For this review, use the dimensioned drawing (mm, ordinates from the lowest corner) and the shaded views. A direction names the side the tool comes from. Coordinates: 2 decimals unless noted, no trailing zeros. Loops run counter-clockwise (first coordinate to the right, second up) from the corner with the lowest first, then second, coordinate; pieces in that order, holes last. Notation, with made-up numbers: (-29.5, 60) - (29.5, 60) arc R18 ccw to (29.5, 70) - close; hole circle Ø4 at (-21, 66). An arc over 180 degrees is marked (long way). Answer in a Markdown table with one row per item. Add a question column.
(1) For P1, Ø4.5, axis at x = 27.432, y = 15.748, coming from the -Z side; P2, Ø6, axis at x = 11.5, z = 5, coming from the +Y side; P3, Ø5, axis at x = 24.5, y = 14, coming from the -Z side; P4, Ø4, axis at x = 9.5, z = 2.5, coming from the +Y side, all flat-tipped, find the tip position at first contact; note any pin that passes through.
(2) For line 1 along X through (y, z) = (12, 9.75); line 2 along X through (y, z) = (7, 2.25); line 3 along Y through (x, z) = (20, 8.5), list the stretches that pass through material, from the lowest coordinate up.
(3) We need section D-D on y = 25. Write out the cut boundary in (x, z) (3 decimals).
(4) Machinability: for the marked faces 5 and 6, which of the approach directions +Z, -Z, +X, -X, +Y, -Y give a long, thin tool a straight path to every point of the face, cutting with its end or side? Answer none if there is none.
(5) Mouldability with a two-part tool opening along Y and no side actions: class the marked faces 1, 2, 3 and 4 as +Y half, -Y half, draft (parallel to the pull), parting line (faces both ways), or undercut.
(6) We need section C-C on x = 2. Write out the cut boundary in (y, z) (3 decimals).
(7) We need section A-A on y = 18.5. Write out the cut boundary in (x, z) (3 decimals), plus the area to 3 significant figures.
(8) We need section B-B on z = 4.75. Write out the cut boundary in (x, y), plus the area to 3 significant figures.
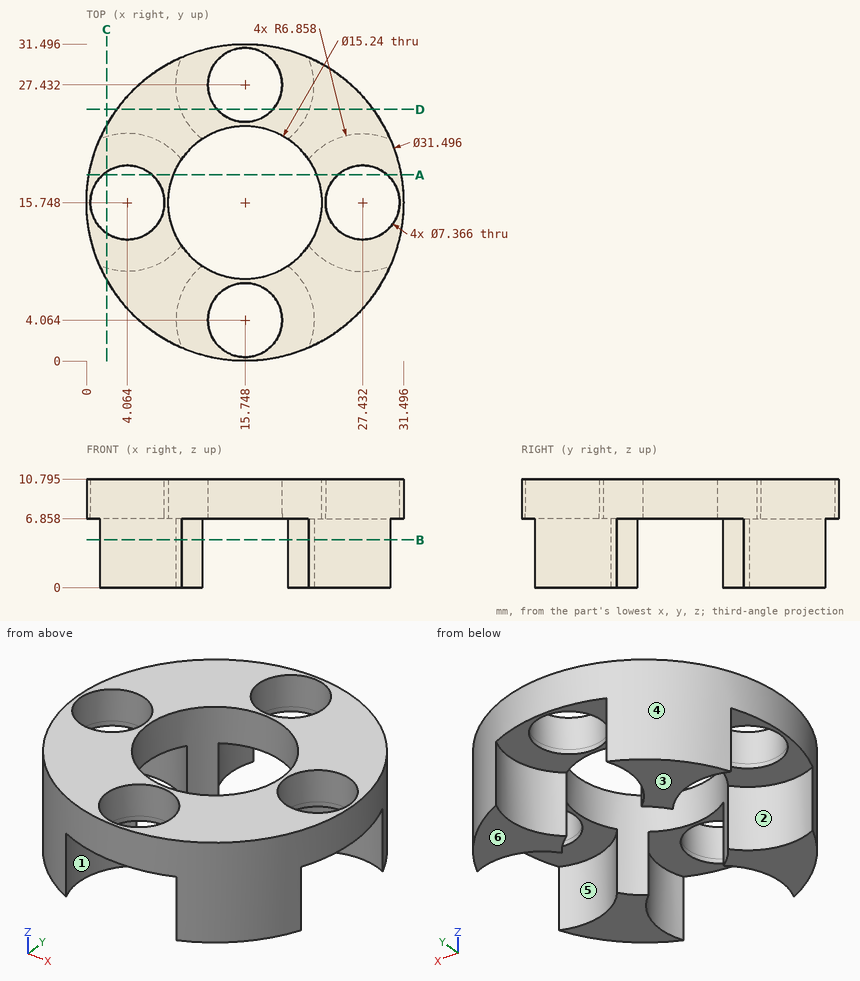
Outcome:
| question | item | result |
|---|---|---|
| 1 | P1 | through |
| 1 | P2 | y = 31.38 |
| 1 | P3 | z = 6.86 |
| 1 | P4 | y = 30.19 |
| 2 | line 1 | 0.45 to 9.11, 22.38 to 31.04 |
| 2 | line 2 | 2.65 to 9.55, 21.95 to 28.84 |
| 2 | line 3 | 0.58 to 9.42, 22.07 to 30.91 |
| 3 | outline | (3.004, 0) - (9.336, 0) - (9.336, 6.858) - (12.982, 6.858) - (12.982, 10.795) - (3.004, 10.795) - close; (18.514, 6.858) - (22.16, 6.858) - (22.16, 0) - (28.492, 0) - (28.492, 10.795) - (18.514, 10.795) - close |
| 4 | face 5 | -Z |
| 4 | face 6 | -Z, +X, -X, +Y, -Y |
| 5 | face 1 | undercut |
| 5 | face 2 | undercut |
| 5 | face 3 | draft |
| 5 | face 4 | parting line |
| 6 | outline | (8.067, 0) - (9.208, 0) - (9.208, 6.858) - (12.698, 6.858) - (12.698, 10.795) - (8.067, 10.795) - close; (18.798, 6.858) - (22.288, 6.858) - (22.288, 0) - (23.429, 0) - (23.429, 10.795) - (18.798, 10.795) - close |
| 7 | outline | (0.242, 6.858) - (1.616, 6.858) - (1.616, 10.795) - (0.242, 10.795) - close; (6.512, 6.858) - (8.642, 6.858) - (8.642, 10.795) - (6.512, 10.795) - close; (22.854, 6.858) - (24.984, 6.858) - (24.984, 10.795) - (22.854, 10.795) - close; (29.88, 6.858) - (31.254, 6.858) - (31.254, 10.795) - (29.88, 10.795) - close |
| 7 | area | 27.6 mm² |
| 8 | outline | (1.31, 9.47) arc R15.75 ccw to (9.47, 1.31) arc R6.86 cw to (11.48, 9.43) arc R7.62 cw to (9.43, 11.48) arc R6.86 cw to start; (1.31, 22.03) arc R6.86 cw to (9.43, 20.01) arc R7.62 cw to (11.48, 22.06) arc R6.86 cw to (9.47, 30.19) arc R15.75 ccw to start; (20.01, 9.43) arc R6.86 cw to (22.03, 1.31) arc R15.75 ccw to (30.19, 9.47) arc R6.86 cw to (22.06, 11.48) arc R7.62 cw to start; (20.01, 22.06) arc R7.62 cw to (22.06, 20.01) arc R6.86 cw to (30.19, 22.03) arc R15.75 ccw to (22.03, 30.19) arc R6.86 cw to start |
| 8 | area | 175 mm² |
